Work out the finished part from the listing and answer in its coordinate system (mm). A direction names the side the tool comes from. Round coordinates to 2 decimals unless told otherwise and drop trailing zeros. Order: outer loops, then holes, each group sorted by start corner. A loop starts at its lowest first (then second) coordinate and runs counter-clockwise, first axis right, second up. Notation, with made-up numbers: M 72.5,61.5 L 82.5,61.5 A20 ccw 82.5,97.5 Z; hole C 81,51.25 d3. An arc over 180 degrees is marked long. Return JSON: item names as keys, results as strings.
from build123d import *

# Parameters (mm, degrees)
SKETCH_R        = 6.3
PAD_DEPTH       = 40
SKETCH001_R     = 4.3
PAD001_DEPTH    = 6
SKETCH002_W     = 1.8
SKETCH002_H     = 1.7
SKETCH002_W_2   = 1.4
SKETCH002_H_2   = 1.9
SKETCH002_W_3   = 1.7
POCKET_DEPTH    = 5.99
SKETCH003_R     = 4.5
POCKET001_DEPTH = 7
SKETCH004_W     = 1.3
SKETCH004_H     = 1.5
SKETCH004_W_2   = 1.5
SKETCH004_H_2   = 1.3
PAD002_DEPTH    = 7
SKETCH005_R     = 1.5
POCKET002_DEPTH = 50


with BuildPart() as part:
    # Sketch → Pad (new body)
    with BuildSketch(Plane.XY):
        with Locations((7, 7)):
            Circle(SKETCH_R)
    extrude(amount=PAD_DEPTH)

    # Sketch001 (on Face3 of Pad) → Pad001 (join)
    with BuildSketch(Plane.XY.offset(40)):
        with Locations((7, 7)):
            Circle(SKETCH001_R)
    extrude(amount=PAD001_DEPTH)

    # Sketch002 (on Face5 of Pad001) → Pocket (cut)
    with BuildSketch(Plane.XY.offset(46)):
        with Locations((7, 11.15)):
            Rectangle(SKETCH002_W, SKETCH002_H)
        with Locations((7, 2.85)):
            Rectangle(SKETCH002_W, SKETCH002_H)
        with Locations((3, 7.05)):
            Rectangle(SKETCH002_W_2, SKETCH002_H_2)
        with Locations((11.15, 7.05)):
            Rectangle(SKETCH002_W_3, SKETCH002_H_2)
    extrude(amount=-POCKET_DEPTH, mode=Mode.SUBTRACT)

    # Sketch003 (on Face2 of Pocket) → Pocket001 (cut)
    with BuildSketch(Plane(origin=(0, 0, 0), x_dir=(1, 0, 0), z_dir=(0, 0, -1))):
        with Locations((7, -7)):
            Circle(SKETCH003_R)
    extrude(amount=-POCKET001_DEPTH, mode=Mode.SUBTRACT)

    # Sketch004 (on Face6 of Pocket001) → Pad002 (join)
    with BuildSketch(Plane(origin=(0, 0, 7), x_dir=(1, 0, 0), z_dir=(0, 0, -1))):
        with Locations((7, -2.9)):
            Rectangle(SKETCH004_W, SKETCH004_H)
        with Locations((7, -11.1)):
            Rectangle(SKETCH004_W, SKETCH004_H)
        with Locations((11.1, -7)):
            Rectangle(SKETCH004_W_2, SKETCH004_H_2)
        with Locations((2.9, -7)):
            Rectangle(SKETCH004_W_2, SKETCH004_H_2)
    extrude(amount=PAD002_DEPTH)

    # Sketch005 (on Face28 of Pad002) → Pocket002 (cut)
    with BuildSketch(Plane.XY.offset(46)):
        with Locations((7, 7)):
            Circle(SKETCH005_R)
    extrude(amount=-POCKET002_DEPTH, mode=Mode.SUBTRACT)


solid = part.part
Item 1: Find section D-D (z = 35). Determine the outline of the cut face in (x, y).
Output:
{"outline": "C 7,7 d12.6; hole C 7,7 d3"}
Item 2: Find section C-C (y = 5). Determine the outline of the cut face in (x, z).
Output:
{"outline": "M 1.03,0 L 2.97,0 L 2.97,7 L 11.03,7 L 11.03,0 L 12.97,0 L 12.97,40 L 10.81,40 L 10.81,46 L 3.19,46 L 3.19,40 L 1.03,40 Z"}
Item 3: Which of the six approach directions +Z, -Z, +X, -X, +Y, -Y give full straight-line access (tool end or side, diameter ignored) to faces 1 (the flat face through (7, 3, 40.01)), 2 (the flat face through (3, 6.1, 43)), 3 (the flat face through (7, 11, 40.01))?
Output:
{"face 1": "+Z, -Y", "face 2": "+Z, -X", "face 3": "+Z, +Y"}
Item 4: Consider line 1 along Y through (x, z) = (7, 27.5); line 2 along Z through (x, y) = (10, 4.5); line 3 along Y through (x, z) = (10, 6). Determine where each line is inside the solid, lowest interval first. Write a range as [from, to].
Output:
{"line 1": "y = [0.7, 5.5], [8.5, 13.3]", "line 2": "z = [7, 46]", "line 3": "y = [1.46, 3.65], [10.35, 12.54]"}
Item 5: The mould has two halves that part along Y. Classify faces 4 (the flat face through (10.35, 7, 4)), 5 (the flat face through (6.1, 3, 43)), 6 (the flat face through (11, 7, 40.01)), 7 (the cylindrical face through (13.01, 8.89, 19.72)): pulls with the +Y half, pulls with the -Y half, needs draft (parallel to the pull), parting line crosses it, or undercut.
Output:
{"face 4": "undercut", "face 5": "needs draft", "face 6": "undercut", "face 7": "parting line crosses it"}
Item 6: Each of these flat-tipped pins is pushed along its axis until it touches: pin 1 (1 mm diameter, centred on y = 8, z = 31.5, fed in from -X); pin 2 (0.6 mm diameter, centred on y = 10.5, z = 2.5, fed in from +X); pin 3 (0.5 mm diameter, centred on y = 10.5, z = 44, fed in from +X). Where does it stop, or does it pass through?
Output:
{"pin 1": "stops at x = 0.72", "pin 2": "stops at x = 12.43", "pin 3": "stops at x = 9.82"}
